Part print with two shaded views. Sizes in mm from the minimum x, y, z corner. Coordinates: 2 decimals unless noted, no trailing zeros. Order: outer loops, then holes, each group sorted by start corner. A loop starts at its lowest first (then second) coordinate and runs counter-clockwise, first axis right, second up. Notation, with made-up numbers: (23.25, 27) - (58.25, 27) arc R33 ccw to (58.25, 62) - close; hole circle Ø3 at (3, 60). An arc over 180 degrees is marked (long way). Write each question's results on one line, items separated by ' | '. Start each with the question number.
Q1. Band-saw the part on A-A, the plane x = 3.6. Write the cut outline in (y, z).
Q2. Wall check: probe 1 along Z at (x, y) = (1.8, 3.35); probe 2 along X at (y, z) = (1.9, 8.5); probe 3 along X at (y, z) = (2.6, 3.25). Give the ranges that are in metal, low to high.
Q3. Pin check, flat tip, straight feed: P1, Ø1.5, axis at x = 2.5, y = 3, coming from the -Z side. Stop position of the tip, or through.
Q4. Band-saw the part on B-B, the plane y = 2.95. Write the cut outline in (x, z) (1 decimal).
Q5. Band-saw the part on D-D, the plane x = 2.45. Write the cut outline in (y, z).
Q6. Band-saw the part on C-C, the plane z = 4. Write the cut outline in (x, y), then the cut area to 3 significant figures.
Q7. Pull direction Z, two halves, no side cores. Call the marked faces 1, 2 and 3: released by +Z, released by -Z, zero draft, split by the parting line, or undercut.
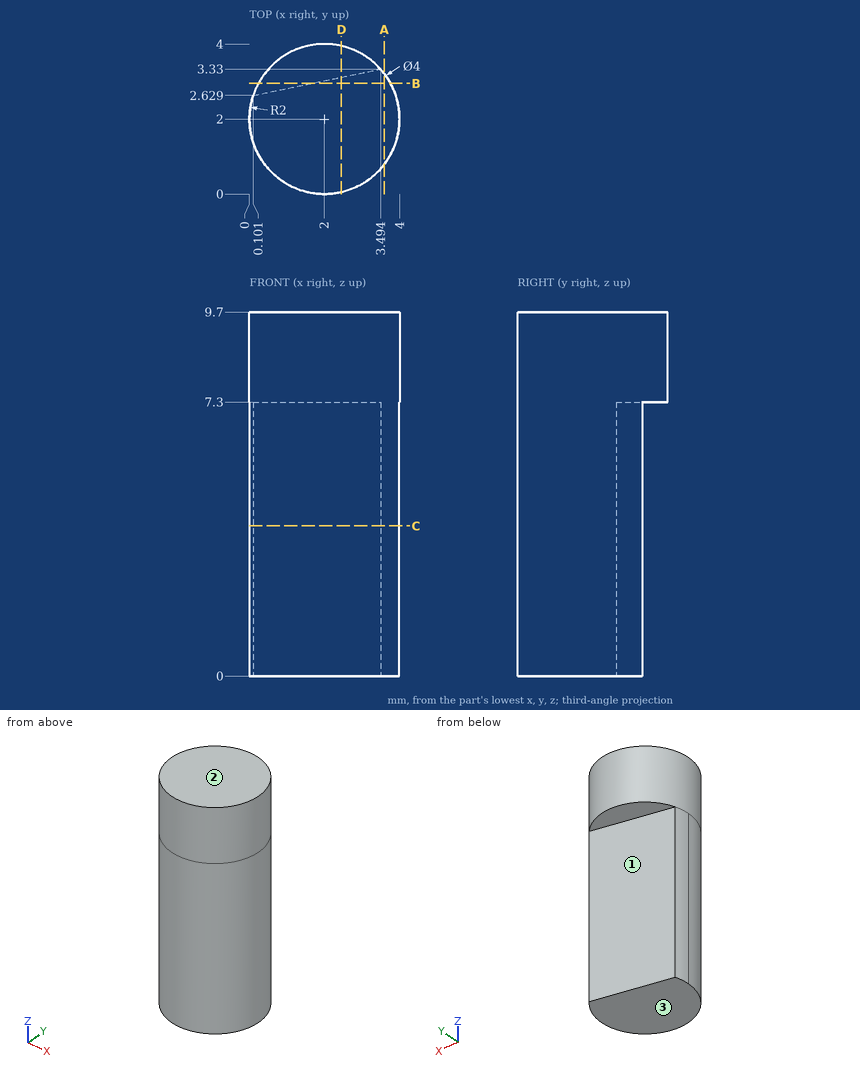
Results below:
1) outline: (0.8, 0) - (3.2, 0) - (3.2, 9.7) - (0.8, 9.7) - close
2) probe 1: z = 7.3 to 9.7 | probe 2: x = 0 to 4 | probe 3: x = 0.09 to 3.91
3) P1: stops at z = 0
4) outline: (0.2, 7.3) - (1.7, 7.3) - (1.7, 0) - (3.8, 0) - (3.8, 9.7) - (0.2, 9.7) - close
5) outline: (0.05, 0) - (3.11, 0) - (3.11, 7.3) - (3.95, 7.3) - (3.95, 9.7) - (0.05, 9.7) - close
6) outline: (0.1, 2.63) arc R2 ccw (long way) to (3.49, 3.33) - close | area: 10.1 mm²
7) face 1: zero draft | face 2: released by +Z | face 3: released by -Z
